Part model, mm, in its own coordinate system. Face numbers are marked on the shaded views. A direction names the side the tool comes from. Round coordinates to 2 decimals unless told otherwise and drop trailing zeros. Loops run counter-clockwise (first coordinate to the right, second up) from the corner with the lowest first, then second, coordinate; pieces in that order, holes last. Notation, with made-up numbers: (68.5, -18.75) -> (75.5, -18.75) arc R20 cw to (75.5, 6.25) -> close; hole circle Ø10 at (74, 6). An arc over 180 degrees is marked (long way). Answer as CSV lines item,"result".
from build123d import *

# Parameters (mm, degrees)
F0_W     = 10
F0_H     = 40
F1_DEPTH = 50
F2_W     = 16.5
F2_H     = 25
F3_DEPTH = 85
F4_R     = 5


with BuildPart() as f1:
    # F0 (on Front) → F1 (new body)
    with BuildSketch(Plane.XZ):
        Polygon((-100, 0), (0, 0), (0, 5), (-10, 5), (-100, 5), align=None)
        Polygon((-10, 45), (0, 45), (0, 50), (-100, 50), (-100, 45), align=None)
        with Locations((-5, 25)):
            Rectangle(F0_W, F0_H)
    extrude(amount=F1_DEPTH)

    # F2 (on Right) → F3 (cut)
    with BuildSketch(Plane.YZ):
        with Locations((-24.75, 12.5)):
            Rectangle(F2_W, F2_H)
    extrude(amount=-F3_DEPTH, mode=Mode.SUBTRACT)

    # F4
    f4_edges = [f1.edges().sort_by_distance(p)[0] for p in [
        (-10, -8.25, 5),
        (-10, -41.5, 5),
        (-10, -25, 45),
    ]]
    fillet(f4_edges, radius=F4_R)


solid = f1.part
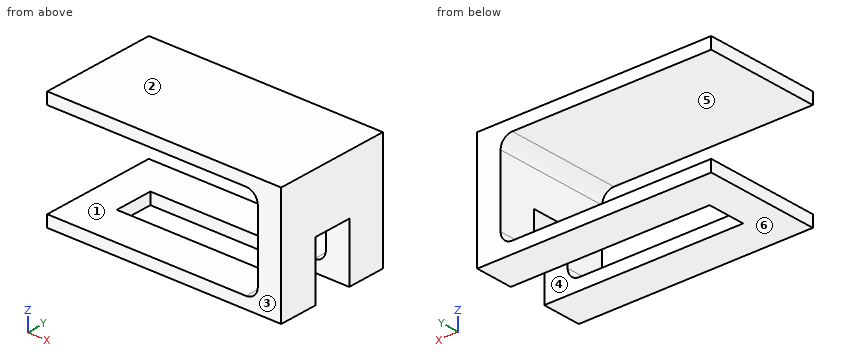
Q1. Drill centre lines: line 1 along Z through (x, y) = (-17, -34); line 2 along Z through (x, y) = (-74.5, -27); line 3 along X through (y, z) = (-26, 39). Where is each one in solid material? Low to high.
Geometry results:
line 1,"0 to 5, 45 to 50"
line 2,"45 to 50"
line 3,"-10 to 0"
Q2. Saw through at D-D, the plane x = -92. Write the cut outline in (y, z), then the cut area to 3 significant figures.
Geometry results:
outline,"(-50, 0) -> (0, 0) -> (0, 5) -> (-50, 5) -> close; (-50, 45) -> (0, 45) -> (0, 50) -> (-50, 50) -> close"
area,"500 mm2"
Q3. Drop flat-ended pins along their axis: P1, Ø12, axis at y = -27, z = 25, coming from the -X side; P2, Ø15, axis at x = -76, y = -19, coming from the -Z side; P3, Ø1.5, axis at y = -22.5, z = 3.5, coming from the +X side. Give the stop position or say it passes through.
Geometry results:
P1,"x = -10"
P2,"z = 0"
P3,"x = -85"
Q4. Which spindle directions (+Z, -Z, +X, -X, +Y, -Y) get a long thin tool onto all of the face, cutting with end or side? Do the marked faces 4, 5 and 6. Say none if no direction does.
Geometry results:
face 4,"-Z, +X"
face 5,"-X, +Y, -Y"
face 6,"-Z, +X, -X, +Y, -Y"
Q5. Saw through at A-A, the plane x = -71.5. Write the cut outline in (y, z), then the cut area to 4 significant figures.
Geometry results:
outline,"(-50, 0) -> (-33, 0) -> (-33, 5) -> (-50, 5) -> close; (-50, 45) -> (0, 45) -> (0, 50) -> (-50, 50) -> close; (-16.5, 0) -> (0, 0) -> (0, 5) -> (-16.5, 5) -> close"
area,"417.5 mm2"
Q6. Saw through at C-C, the plane y = -45. Write the cut outline in (x, z), then the cut area to 3 significant figures.
Geometry results:
outline,"(-100, 0) -> (0, 0) -> (0, 50) -> (-100, 50) -> (-100, 45) -> (-15, 45) arc R5 cw to (-10, 40) -> (-10, 10) arc R5 cw to (-15, 5) -> (-100, 5) -> close"
area,"1,410 mm2"
Q7. Two-plate mould, pull along Z, no slides. Class the marked faces 1, 2 and 3: pulls with the +Z half, pulls with the -Z half, needs draft (parallel to the pull), parting line crosses it, or undercut.
Geometry results:
face 1,"undercut"
face 2,"pulls with the +Z half"
face 3,"needs draft"
Q8. Saw through at B-B, the plane z = 14. Write the cut outline in (x, y).
Geometry results:
outline,"(-10, -50) -> (0, -50) -> (0, -33) -> (-10, -33) -> close; (-10, -16.5) -> (0, -16.5) -> (0, 0) -> (-10, 0) -> close"
